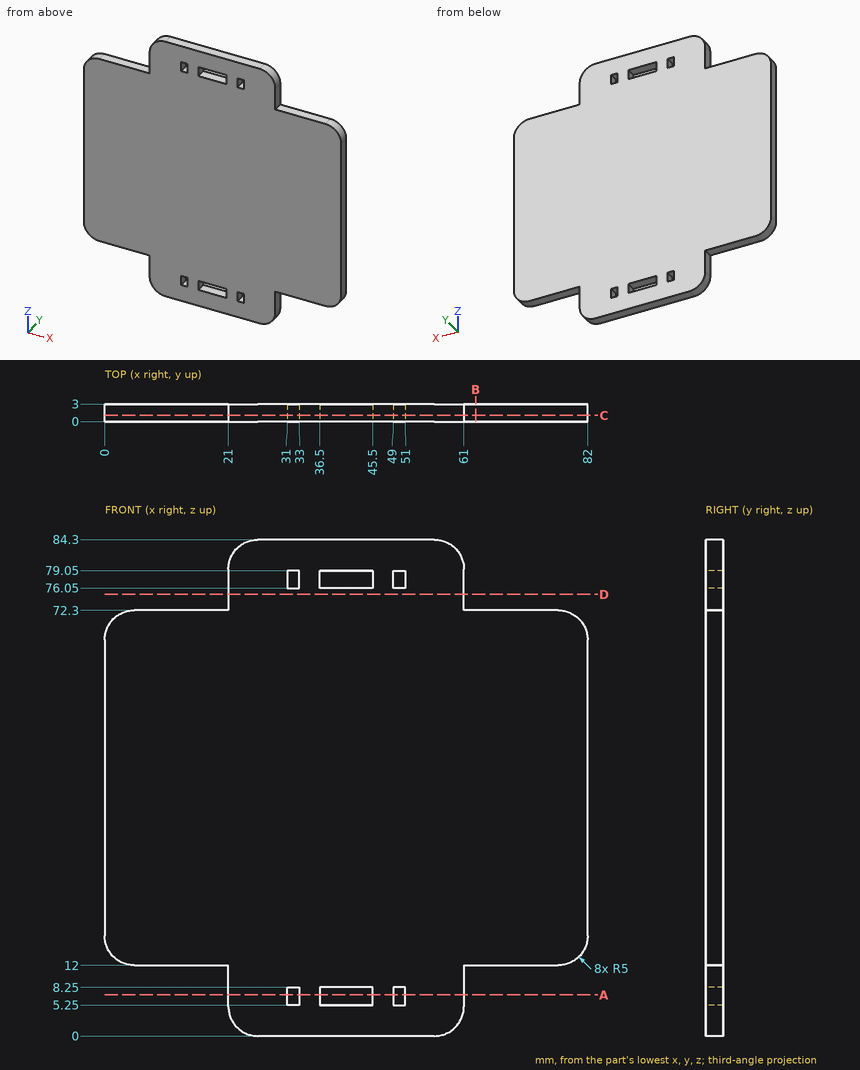
Could you check a few things on this drawing? It's one solid part, dimensions in mm from its lowest x, y, z. Round coordinates to 2 decimals unless told otherwise and drop trailing zeros. Order: outer loops, then holes, each group sorted by start corner. A loop starts at its lowest first (then second) coordinate and runs counter-clockwise, first axis right, second up. Notation, with made-up numbers: M 55,79.25 L 70,79.25 A26 ccw 70,108.25 Z; hole C -15,-15.75 d6. An arc over 180 degrees is marked long. Return JSON: item names as keys, results as strings. Group by question number.
1. If we section it at C-C on y = 1.05: State how many separate pieces and enclosed holes the cut face has, then the cut area to 3 significant figures.
2. I'm going to push flat-ended pins straight in: pin 1 Ø1 at (x, y) = (14.5, 2) entering from -Z; pin 2 Ø1 at (x, z) = (10.5, 40) entering from -Y; pin 3 Ø0.9 at (y, z) = (2, 8) entering from +X; pin 4 Ø1.5 at (x, y) = (72, 2) entering from +Z. Where does each tip first touch, or does it pass through?
3. If we section it at D-D on z = 75: List the corners of the cut face in (x, y) for me, then the cut area to 3 significant figures.
4. If we section it at B-B on x = 63: List the corners of the cut face in (y, z) for me, then the cut area to 3 significant figures.
5. Please list where these lines run through material, in increasing order: probe 1 along Z at (x, y) = (18, 2.5); probe 2 along X at (y, z) = (0.25, 76); probe 3 along X at (y, z) = (2.35, 16).
6. If we section it at A-A on z = 7: List the corners of the cut face in (x, y) for me.
Reply:
{
 "1": {"separate pieces": "1", "enclosed holes": "6", "area": "5,780 mm^2"},
 "2": {"pin 1": "z = 12", "pin 2": "y = 0", "pin 3": "x = 61", "pin 4": "z = 72.3"},
 "3": {"outline": "M 21,0 L 61,0 L 61,3 L 21,3 Z", "area": "120 mm^2"},
 "4": {"outline": "M 0,12 L 3,12 L 3,72.3 L 0,72.3 Z", "area": "181 mm^2"},
 "5": {"probe 1": "12 to 72.3", "probe 2": "21 to 61", "probe 3": "0.1 to 81.9"},
 "6": {"outline": "M 21,0 L 31,0 L 31,3 L 21,3 Z; M 33,0 L 36.5,0 L 36.5,3 L 33,3 Z; M 45.5,0 L 49,0 L 49,3 L 45.5,3 Z; M 51,0 L 61,0 L 61,3 L 51,3 Z"}
}
